Part model, mm, in its own coordinate system. Face numbers are marked on the shaded views. Coordinates: 2 decimals unless noted, no trailing zeros. Order: outer loops, then holes, each group sorted by start corner. A loop starts at its lowest first (then second) coordinate and runs counter-clockwise, first axis right, second up.
1) Cut at D-D (z = 1.65). Give the number of separate pieces and of enclosed holes in the cut face, and give its area (3 significant figures).
2) Cut at C-C (y = 27). List the corners of the cut face in (x, z).
3) Cut at B-B (y = 18.5). List the corners of the cut face in (x, z).
4) Pin check, flat tips, straight feed: pin 1 Ø2 at (x, z) = (17, 3) entering from +Y; pin 2 Ø1.2 at (y, z) = (-2.5, 2) entering from +X; pin 3 Ø1.2 at (y, z) = (-2.5, 4) entering from -X. Stop position of each tip, or through.
5) Wall check: L1, parallel to X at y = -2, z = 0.35; L2, parallel to Y at x = 99.5, z = 4.5; L3, parallel to X at y = 27, z = 2.65. Give the ranges that are in metal, low to high.
6) Cut at A-A (x = 99.5). List the corners of the cut face in (y, z).
7) Mould opens along X. For the marked faces 1 and 2 say: +X half, -X half, draft (parallel to the pull), parting line (faces both ways), or undercut.
Autodesk Inventor part; units mm, degrees
ref_plane "YZ Plane" through (0, 0, 0) normal (1, 0, 0) x (0, 1, 0)
ref_plane "XZ Plane" through (0, 0, 0) normal (0, 1, 0) x (-1, 0, 0)
ref_plane "XY Plane" through (0, 0, 0) normal (0, 0, 1) x (1, 0, 0)
sketch "Sketch1" plane through (0, 0, 0) normal (0, 0, 1) x (1, 0, 0)
  line L0 (0, 4) -> (0, 0)
  line L1 (0, 0) -> (125, 0)
  line L2 (0, 4) -> (57, 23)
  line L3 (103, 14) -> (103, 8)
  line L4 (103, 8) -> (73, 8)
  line L5 (73, 8) -> (73, 14)
  line L6 (125, 14) -> (121, 14)
  line L7 (121, 14) -> (121, 8)
  line L8 (121, 8) -> (125, 8)
  line L9 (125, 0) -> (125, 8)
  line L10 (125, 14) -> (125, 23)
  line L11 (81, 23) -> (81, 14)
  line L12 (92, 14) -> (92, 23)
  line L13 (73, 14) -> (81, 14)
  line L14 (92, 14) -> (103, 14)
  line L15 (81, 14) -> (92, 14) construction
  circle A0 centre (86.5, 19.099) radius 7.5 construction
  circle A1 centre (86.5, 19.099) radius 4 construction
  line L16 (113.5, 21.4084) -> (113.5, 16.7896)
  line L17 (113.5, 16.7896) -> (109.5, 14.4802)
  line L18 (109.5, 14.4802) -> (105.5, 16.7896)
  line L19 (105.5, 16.7896) -> (105.5, 21.4084)
  line L20 (105.5, 21.4084) -> (109.5, 23.7178)
  line L21 (109.5, 23.7178) -> (113.5, 21.4084)
  circle A2 centre (109.5, 19.099) radius 2.5 construction
  line L22 (105.5, 23) -> (105.5, 29)
  line L23 (107.5, 31) -> (111.5, 31)
  line L24 (113.5, 29) -> (113.5, 23)
  arc A3 (107.5, 31) -> (105.5, 29) centre (107.5, 29) ccw
  arc A4 (113.5, 29) -> (111.5, 31) centre (111.5, 29) ccw
  line L25 (125, 23) -> (113.5, 23)
  line L26 (105.5, 23) -> (92, 23)
  circle A5 centre (99.5, 18.5) radius 4.5 construction
  circle A6 centre (119.5, 18.5) radius 4.5 construction
  circle A7 centre (99.5, 18.5) radius 2.25
  circle A8 centre (119.5, 18.5) radius 2.25
  line L27 (67, 23) -> (67, 29)
  line L28 (69, 31) -> (73, 31)
  line L29 (75, 29) -> (75, 23)
  arc A9 (69, 31) -> (67, 29) centre (69, 29) ccw
  arc A10 (75, 29) -> (73, 31) centre (73, 29) ccw
  line L30 (81, 23) -> (75, 23)
  line L31 (67, 23) -> (57, 23)
  point P0 (81, 14)
  point P1 (92, 14)
  point P2 (86.5, 14)
  point P3 (125, 18.5)
  point P4 (109.5, 31)
  dimension "d0" = 8
  dimension "d2" = 6
  dimension "d3" = 4
  dimension "d4" = 15
  dimension "d5" = 8
  dimension "d6" = 9
  dimension "d7" = 11
  dimension "d8" = 11
  dimension "d9" = 8
  dimension "d10" = 5
  dimension "d11" = 2
  dimension "d12" = 8
  dimension "d13" = 9
  dimension "d14" = 9
  dimension "d15" = 10
  dimension "d16" = 10
  dimension "d17" = 4.5
  dimension "d18" = 4.5
  dimension "d19" = 13
  dimension "d20" = 5.5
  dimension "d21" = 18
  dimension "d22" = 2
  dimension "d23" = 8
  dimension "d24" = 6
  dimension "d25" = 10
  dimension "d27" = 30
  dimension "d28" = 4
  dimension "d30" = 8
  dimension "d31" = 125
extrude "Extrusion1" add sketch "Sketch1" along normal blind 6
sketch "Sketch2" plane through (0, 0, 6) normal (0, 0, 1) x (1, 0, 0)
  line L0 (0, 4) -> (0, 0)
  line L1 (0, 0) -> (125, 0)
  line L2 (6, 0) -> (14, 0)
  line L3 (14, 0) -> (14, -4)
  line L4 (12, -6) -> (8, -6)
  line L5 (6, -4) -> (6, 0)
  line L6 (57, 0) -> (65, 0)
  line L7 (65, 0) -> (65, -4)
  line L8 (63, -6) -> (59, -6)
  line L9 (57, -4) -> (57, 0)
  line L10 (85, 0) -> (93, 0)
  line L11 (93, 0) -> (93, -4)
  line L12 (91, -6) -> (87, -6)
  line L13 (85, -4) -> (85, 0)
  line L14 (113, 0) -> (121, 0)
  line L15 (121, 0) -> (121, -4)
  line L16 (119, -6) -> (115, -6)
  line L17 (113, -4) -> (113, 0)
  arc A0 (6, -4) -> (8, -6) centre (8, -4) ccw
  arc A1 (12, -6) -> (14, -4) centre (12, -4) ccw
  arc A2 (57, -4) -> (59, -6) centre (59, -4) ccw
  arc A3 (63, -6) -> (65, -4) centre (63, -4) ccw
  arc A4 (85, -4) -> (87, -6) centre (87, -4) ccw
  arc A5 (91, -6) -> (93, -4) centre (91, -4) ccw
  arc A6 (113, -4) -> (115, -6) centre (115, -4) ccw
  arc A7 (119, -6) -> (121, -4) centre (119, -4) ccw
  dimension "d34" = 2
  dimension "d35" = 8
  dimension "d36" = 8
  dimension "d37" = 8
  dimension "d38" = 8
  dimension "d39" = 6
  dimension "d40" = 6
  dimension "d41" = 43
  dimension "d42" = 20
  dimension "d43" = 20
extrude "Extrusion2" add sketch "Sketch2" against normal blind 6
sketch "Sketch3" plane through (0, 0, 6) normal (0, 0, 1) x (1, 0, 0)
  line L0 (0, 4) -> (0, 0)
  line L1 (14, 0) -> (57, 0)
  line L2 (30, 0) -> (40, 0)
  line L3 (40, 0) -> (40, 5)
  line L4 (39, 6) -> (31, 6)
  line L5 (30, 5) -> (30, 0)
  arc A0 (31, 6) -> (30, 5) centre (31, 5) ccw
  arc A1 (40, 5) -> (39, 6) centre (39, 5) ccw
  point P0 (35, 6)
  dimension "d46" = 1
  dimension "d47" = 10
  dimension "d48" = 6
  dimension "d49" = 35
extrude "Extrusion3" cut sketch "Sketch3" against normal through all
properties part number "x_motor_wall_lower"
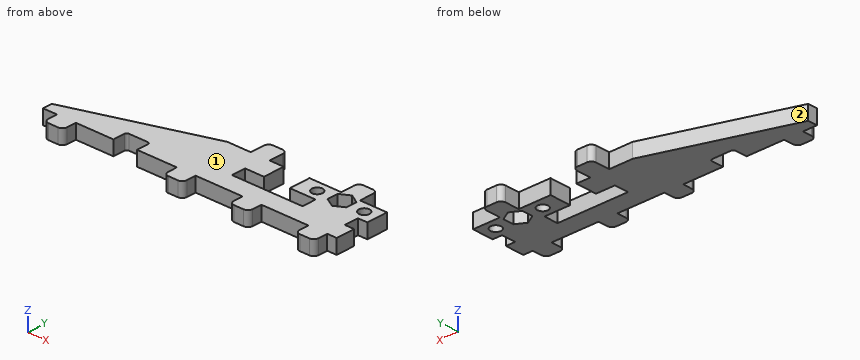
Geometry check:
1. separate pieces: 1
1. enclosed holes: 3
1. area: 2,190 mm2
2. outline: (67, 0) - (75, 0) - (75, 6) - (67, 6) - close; (105.5, 0) - (113.5, 0) - (113.5, 6) - (105.5, 6) - close
3. outline: (43.5, 0) - (81, 0) - (81, 6) - (43.5, 6) - close; (92, 0) - (97.25, 0) - (97.25, 6) - (92, 6) - close; (101.75, 0) - (105.5, 0) - (105.5, 6) - (101.75, 6) - close; (113.5, 0) - (117.25, 0) - (117.25, 6) - (113.5, 6) - close; (121.75, 0) - (125, 0) - (125, 6) - (121.75, 6) - close
4. pin 1: stops at y = 10
4. pin 2: stops at x = 121
4. pin 3: stops at x = 6
5. L1: x = 6 to 14, 57 to 65, 85 to 93, 113 to 121
5. L2: y = 0 to 8, 14 to 16.25, 20.75 to 23
5. L3: x = 67 to 75, 105.5 to 113.5
6. outline: (0, 0) - (8, 0) - (8, 6) - (0, 6) - close; (14, 0) - (16.25, 0) - (16.25, 6) - (14, 6) - close; (20.75, 0) - (23, 0) - (23, 6) - (20.75, 6) - close
7. face 1: draft
7. face 2: -X half
